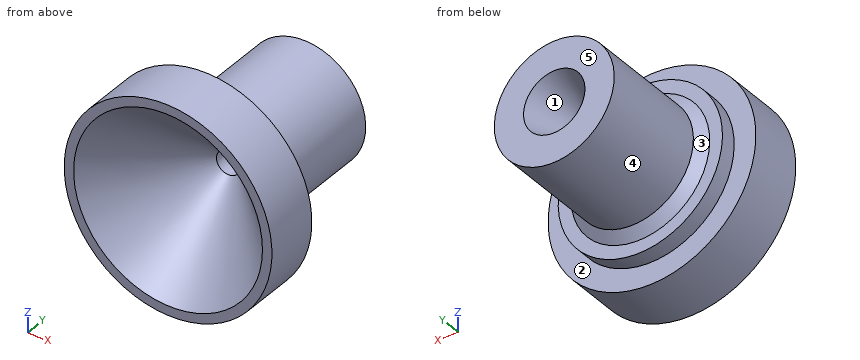
```python
from build123d import *

# Parameters (mm, degrees)
SKETCH1_R           = 11
BOSS_EXTRUDE1_DEPTH = 5.8
SKETCH2_R           = 8.7
BOSS_EXTRUDE2_DEPTH = 1.7
SKETCH3_R           = 6.35
BOSS_EXTRUDE3_DEPTH = 12.5
CHAMFER1_SIZE       = 1
SKETCH4_R           = 1.25
CUT_EXTRUDE1_DEPTH  = 26.337718919
SKETCH5_R           = 3.25
CUT_EXTRUDE2_DEPTH  = 8
CUT_EXTRUDE2_DRAFT  = -20
SKETCH6_R           = 10
CUT_EXTRUDE3_DEPTH  = 9
CUT_EXTRUDE3_DRAFT  = -45


with BuildPart() as part:
    # Sketch1 → Boss-Extrude1 (new body)
    with BuildSketch(Plane(origin=(0, 0, 0), x_dir=(1, 0, 0), z_dir=(0, 1, 0))):
        with Locations(Location((0, 0, 0), (0, 0, 270))):
            Circle(SKETCH1_R)
    extrude(amount=BOSS_EXTRUDE1_DEPTH)

    # Sketch2 → Boss-Extrude2 (add)
    with BuildSketch(Plane(origin=(0, 5.8, 0), x_dir=(1, 0, 0), z_dir=(0, 1, 0))):
        with Locations(Location((0, 0, 0), (0, 0, 270))):
            Circle(SKETCH2_R)
    extrude(amount=BOSS_EXTRUDE2_DEPTH)

    # Sketch3 → Boss-Extrude3 (add)
    with BuildSketch(Plane(origin=(0, 7.5, 0), x_dir=(1, 0, 0), z_dir=(0, 1, 0))):
        with Locations(Location((0, 0, 0), (0, 0, 270))):
            Circle(SKETCH3_R)
    extrude(amount=BOSS_EXTRUDE3_DEPTH)

    # Chamfer1
    chamfer1_edges = [part.edges().sort_by_distance(p)[0] for p in [
        (0, 7.5, -6.35),
    ]]
    chamfer(chamfer1_edges, length=CHAMFER1_SIZE)

    # Sketch4 → Cut-Extrude1 (cut, through all)
    with BuildSketch(Plane(origin=(0, 20, 0), x_dir=(1, 0, 0), z_dir=(0, 1, 0))):
        with Locations(Location((0, 0, 0), (0, 0, 270))):
            Circle(SKETCH4_R)
    extrude(amount=-CUT_EXTRUDE1_DEPTH, mode=Mode.SUBTRACT)


with BuildPart() as cut_extrude2_tool:
    # Sketch5 → Cut-Extrude2 (with draft: the straight prism first)
    with BuildSketch(Plane(origin=(0, 20, 0), x_dir=(1, 0, 0), z_dir=(0, 1, 0))):
        Circle(SKETCH5_R)
    extrude(amount=-CUT_EXTRUDE2_DEPTH)
    # Cut-Extrude2: the draft: its side faces are tilted about the plane it starts from
    cut_extrude2_sides = [cut_extrude2_tool.faces().sort_by_distance(p)[0] for p in [
        (-3.25, 16, 0),
    ]]
    draft(cut_extrude2_sides, Plane(origin=(0, 20, 0), x_dir=(1, 0, 0), z_dir=(0, 1, 0)), CUT_EXTRUDE2_DRAFT)


with BuildPart() as part_1:
    add(part.part)

    # Cut-Extrude2: cut by cut_extrude2_tool
    add(cut_extrude2_tool.part, mode=Mode.SUBTRACT)


with BuildPart() as cut_extrude3_tool:
    # Sketch6 → Cut-Extrude3 (with draft: the straight prism first)
    with BuildSketch(Plane.XZ):
        Circle(SKETCH6_R)
    extrude(amount=-CUT_EXTRUDE3_DEPTH)
    # Cut-Extrude3: the draft: its side faces are tilted about the plane it starts from
    cut_extrude3_sides = [cut_extrude3_tool.faces().sort_by_distance(p)[0] for p in [
        (-10, 4.5, 0),
    ]]
    draft(cut_extrude3_sides, Plane.XZ, CUT_EXTRUDE3_DRAFT)


with BuildPart() as part_2:
    add(part_1.part)

    # Cut-Extrude3: cut by cut_extrude3_tool
    add(cut_extrude3_tool.part, mode=Mode.SUBTRACT)


solid = part_2.part
```
Here's how the part is built. I have some questions about the finished solid (model axes, mm). Face numbers are marked on the shaded views. A direction names the side the tool comes from. Round coordinates to 2 decimals unless told otherwise and drop trailing zeros. Order: outer loops, then holes, each group sorted by start corner. A loop starts at its lowest first (then second) coordinate and runs counter-clockwise, first axis right, second up. Notation, with made-up numbers: (53, 65) -> (79, 65) arc R8 cw to (79, 77) -> close; hole circle Ø6 at (56, 34). An arc over 180 degrees is marked (long way). Use a Markdown table: item, result. Add a question column.
(1) Suppose I cut it at A-A, the plane z = 0. Please give me the cut outline in (x, y), and give its area (3 significant figures).
(2) Suppose I cut it at B-B, the plane x = 0. Please give me the cut outline in (y, z).
(3) For the marked faces 4 and 5, which set-ups out of +Z, -Z, +X, -X, +Y, -Y let a thin tool reach every point of the face, with its end or its side?
(4) Suppose I cut it at C-C, the plane y = 2. Please give me the cut outline in (x, z).
(5) I need wall thicknesses on line 1 along X through (y, z) = (10.7, 0); line 2 along X through (y, z) = (5, -1); line 3 along Z through (x, y) = (2.25, 7). Which ranges of each line are inside material? Lowest first, please.
(6) For pin 1 Ø1 at (y, z) = (13.5, -0.5) entering from -X; pin 2 Ø3 at (x, y) = (6, 14) entering from -Z; pin 3 Ø6 at (y, z) = (3, 8.5) entering from -X, each with a flat end and sliding along its axis, tell me the tip position at first contact or that it passes through.
(7) If we mould it in two halves opening along Z, with no side actions, what happens to the marked faces 1, 2 and 3? For each: released by +Z, released by -Z, zero draft, split by the parting line, or undercut.
(8) Suppose I cut it at D-D, the plane y = 4. Please give me the cut outline in (x, z).
Verdict:
| question | item | result |
|---|---|---|
| 1 | outline | (-11, 0) -> (-10, 0) -> (-1.25, 8.75) -> (-1.25, 14.51) -> (-3.25, 20) -> (-6.35, 20) -> (-6.35, 8.5) -> (-7.35, 7.5) -> (-8.7, 7.5) -> (-8.7, 5.8) -> (-11, 5.8) -> close; (1.25, 8.75) -> (10, 0) -> (11, 0) -> (11, 5.8) -> (8.7, 5.8) -> (8.7, 7.5) -> (7.35, 7.5) -> (6.35, 8.5) -> (6.35, 20) -> (3.25, 20) -> (1.25, 14.51) -> close |
| 1 | area | 179 mm2 |
| 2 | outline | (0, -11) -> (5.8, -11) -> (5.8, -8.7) -> (7.5, -8.7) -> (7.5, -7.35) -> (8.5, -6.35) -> (20, -6.35) -> (20, -3.25) -> (14.51, -1.25) -> (8.75, -1.25) -> (0, -10) -> close; (0, 10) -> (8.75, 1.25) -> (14.51, 1.25) -> (20, 3.25) -> (20, 6.35) -> (8.5, 6.35) -> (7.5, 7.35) -> (7.5, 8.7) -> (5.8, 8.7) -> (5.8, 11) -> (0, 11) -> close |
| 3 | face 4 | +Y |
| 3 | face 5 | +Z, -Z, +X, -X, +Y |
| 4 | outline | circle Ø22 at (0, 0); hole circle Ø16 at (0, 0) |
| 5 | line 1 | -6.35 to -1.25, 1.25 to 6.35 |
| 5 | line 2 | -10.95 to -4.9, 4.9 to 10.95 |
| 5 | line 3 | -8.4 to -1.98, 1.98 to 8.4 |
| 6 | pin 1 | x = -6.35 |
| 6 | pin 2 | z = -4.48 |
| 6 | pin 3 | x = -9.53 |
| 7 | face 1 | undercut |
| 7 | face 2 | zero draft |
| 7 | face 3 | split by the parting line |
| 8 | outline | circle Ø22 at (0, 0); hole circle Ø12 at (0, 0) |
